```python
from build123d import *

# Parameters (mm, degrees)
SKETCH1_R           = 25
BOSS_EXTRUDE1_DEPTH = 5
SKETCH3_R           = 2.5
CUT_EXTRUDE1_DEPTH  = 18


with BuildPart() as part:
    # Sketch1 → Boss-Extrude1 (new body)
    with BuildSketch(Plane(origin=(0, 0, 0), x_dir=(1, 0, 0), z_dir=(0, 1, 0))):
        with Locations(Location((0, 0, 0), (0, 0, 270))):
            Circle(SKETCH1_R)
        Polygon((-9.872689603, 0), (-4.936344802, -8.55), (4.936344802, -8.55), (9.872689603, 0), (4.936344802, 8.55), (-4.936344802, 8.55), align=None, mode=Mode.SUBTRACT)
    extrude(amount=BOSS_EXTRUDE1_DEPTH)

    # Sketch3 → Cut-Extrude1 (cut)
    with BuildSketch(Plane(origin=(0, 5, 0), x_dir=(1, 0, 0), z_dir=(0, 1, 0))):
        with Locations(Location((0, 17.5, 0), (0, 0, 270))):
            Circle(SKETCH3_R)
        with Locations(Location((17.5, 0, 0), (0, 0, 270))):
            Circle(SKETCH3_R)
        with Locations(Location((0, -17.5, 0), (0, 0, 270))):
            Circle(SKETCH3_R)
        with Locations(Location((-17.5, 0, 0), (0, 0, 270))):
            Circle(SKETCH3_R)
    extrude(amount=-CUT_EXTRUDE1_DEPTH, mode=Mode.SUBTRACT)


solid = part.part
```
Can you work these out from the model? Positions are in its coordinate system, mm. A direction names the side the tool comes from. Round coordinates to 2 decimals unless told otherwise and drop trailing zeros. Loops run counter-clockwise (first coordinate to the right, second up) from the corner with the lowest first, then second, coordinate; pieces in that order, holes last. Notation, with made-up numbers: (-12.5, 87.5) -> (25.5, 87.5) arc R27 ccw to (25.5, 106.5) -> close; hole circle Ø7 at (58.5, 48.25). An arc over 180 degrees is marked (long way). One line per item, written item: value. Start each with the question number.
1. If we section it at D-D, the plane x = -17.5: Write out the boundary of the cut face in (y, z).
2. If we section it at B-B, the plane z = -16: Write out the boundary of the cut face in (x, y), then the cut area to 3 significant figures.
3. For pin 1 (2 mm diameter, centred on x = 13, y = 3.5, fed in from -Z); pin 2 (2.5 mm diameter, centred on x = 1.5, y = 2, fed in from +Z); pin 3 (1.5 mm diameter, centred on y = 1.5, z = 20, fed in from -X); pin 4 (4.5 mm diameter, centred on x = 17.5, z = 0, fed in from +Y), each with a flat end and sliding along its axis, tell me the tip position at first contact or that it passes through.
4. If we section it at A-A, the plane x = 0: Write out the boundary of the cut face in (y, z).
5. For faces 1 (the flat face through (-11, 0, 0)), 2 (the flat face through (-7.439, 2.465, 4.215)), which set-ups out of +Z, -Z, +X, -X, +Y, -Y let a thin tool reach every point of the face, with its end or its side?
6. If we mould it in two halves opening along X, with no side actions, what happens to faces 3 (the flat face through (-11, 5, 0)), 4 (the cylindrical face through (7.509, 2.465, 23.846)), 5 (the flat face through (0, 2, 8.55))? For each: pulls with the +X half, pulls with the -X half, needs draft (parallel to the pull), parting line crosses it, or undercut.
7. If we section it at C-C, the plane y = 3.75: Write out the boundary of the cut face in (x, z).
8. If I drill on probe 1 along X at (y, z) = (2.25, 0); probe 2 along X at (y, z) = (2.15, 1); probe 3 along Z at (x, y) = (-16.5, 2.4), over which ranges is the centre line in solid material (lowest first)?
Calculated:
1. outline: (0, -17.85) -> (5, -17.85) -> (5, -2.5) -> (0, -2.5) -> close; (0, 2.5) -> (5, 2.5) -> (5, 17.85) -> (0, 17.85) -> close
2. outline: (-19.21, 0) -> (-2, 0) -> (-2, 5) -> (-19.21, 5) -> close; (2, 0) -> (19.21, 0) -> (19.21, 5) -> (2, 5) -> close
2. area: 172 mm²
3. pin 1: stops at z = -21.93
3. pin 2: stops at z = 25
3. pin 3: stops at x = -15.95
3. pin 4: passes through
4. outline: (0, -25) -> (5, -25) -> (5, -20) -> (0, -20) -> close; (0, -15) -> (5, -15) -> (5, -8.55) -> (0, -8.55) -> close; (0, 8.55) -> (5, 8.55) -> (5, 15) -> (0, 15) -> close; (0, 20) -> (5, 20) -> (5, 25) -> (0, 25) -> close
5. face 1: +Z, -Z, +X, -X, -Y
5. face 2: +Y, -Y
6. face 3: needs draft
6. face 4: parting line crosses it
6. face 5: undercut
7. outline: circle Ø50 at (0, 0); hole circle Ø5 at (-17.5, 0); hole (-9.87, 0) -> (-4.94, -8.55) -> (4.94, -8.55) -> (9.87, 0) -> (4.94, 8.55) -> (-4.94, 8.55) -> close; hole circle Ø5 at (0, -17.5); hole circle Ø5 at (0, 17.5); hole circle Ø5 at (17.5, 0)
8. probe 1: x = -25 to -20, -15 to -9.87, 9.87 to 15, 20 to 25
8. probe 2: x = -24.98 to -19.79, -15.21 to -9.3, 9.3 to 15.21, 19.79 to 24.98
8. probe 3: z = -18.78 to -2.29, 2.29 to 18.78
